from build123d import *

# Parameters (mm, degrees)
SKETCH1_W            = 210
SKETCH1_H            = 210
BASE_DEPTH           = 4
WALLS_START          = 4
SKETCH1_3_W          = 210
SKETCH1_3_H          = 210
SKETCH1_3_W_2        = 202
SKETCH1_3_H_2        = 202
WALLS_DEPTH          = 25.4
SCREWMOUNTS_DEPTH    = 25.4
SKETCH2_5_R          = 1.5
SCREWHOLES_DEPTH     = 12.5
ROUNDEDCORNERS_R     = 10
BACKHOLEMOUNTS_DEPTH = 4
SKETCH4_R            = 1.5
SKETCH4_W            = 30
SKETCH4_H            = 10
BATTERYPACK_DEPTH    = 4


with BuildPart() as part:
    # Sketch1 → Base (new body)
    with BuildSketch(Plane(origin=(0, 0, 0), x_dir=(1, 0, 0), z_dir=(0, 1, 0))):
        Rectangle(SKETCH1_W, SKETCH1_H)
    extrude(amount=BASE_DEPTH)

    # Sketch1<3> → Walls (add)
    with BuildSketch(Plane(origin=(0, 0, 0), x_dir=(1, 0, 0), z_dir=(0, 1, 0)).offset(WALLS_START)):
        Rectangle(SKETCH1_3_W, SKETCH1_3_H)
        Rectangle(SKETCH1_3_W_2, SKETCH1_3_H_2, mode=Mode.SUBTRACT)
    extrude(amount=WALLS_DEPTH)

    # Sketch2 → ScrewMounts (add)
    with BuildSketch(Plane(origin=(0, 29.4, 0), x_dir=(1, 0, 0), z_dir=(0, 1, 0))):
        with BuildLine():
            Line((-101, 101), (-101, 96))
            ThreePointArc((-101, 96), (-97.464466094, 97.464466094), (-96, 101))
            Line((-96, 101), (-101, 101))
        make_face()
        with BuildLine():
            Line((-101, -101), (-96, -101))
            ThreePointArc((-96, -101), (-97.464466094, -97.464466094), (-101, -96))
            Line((-101, -96), (-101, -101))
        make_face()
        with BuildLine():
            Line((101, 101), (96, 101))
            ThreePointArc((96, 101), (97.464466094, 97.464466094), (101, 96))
            Line((101, 96), (101, 101))
        make_face()
        with BuildLine():
            Line((101, -101), (101, -96))
            ThreePointArc((101, -96), (97.464466094, -97.464466094), (96, -101))
            Line((96, -101), (101, -101))
        make_face()
    extrude(amount=-SCREWMOUNTS_DEPTH)

    # Sketch2<5> → ScrewHoles (cut)
    with BuildSketch(Plane(origin=(0, 29.4, 0), x_dir=(1, 0, 0), z_dir=(0, 1, 0))):
        with Locations((-99.833273811, 99.833273811)):
            Circle(SKETCH2_5_R)
        with Locations((-99.833273811, -99.833273811)):
            Circle(SKETCH2_5_R)
        with Locations((99.833273811, 99.833273811)):
            Circle(SKETCH2_5_R)
        with Locations((99.833273811, -99.833273811)):
            Circle(SKETCH2_5_R)
    extrude(amount=-SCREWHOLES_DEPTH, mode=Mode.SUBTRACT)

    # RoundedCorners
    roundedcorners_edges = [part.edges().sort_by_distance(p)[0] for p in [
        (-105, 14.7, 105),
        (105, 14.7, 105),
        (105, 14.7, -105),
        (-105, 14.7, -105),
    ]]
    fillet(roundedcorners_edges, radius=ROUNDEDCORNERS_R)

    # Sketch3 → BackHoleMounts (cut)
    with BuildSketch(Plane.XZ):
        with BuildLine():
            Line((-77.985, 80), (-77.985, 61.974012195))
            ThreePointArc((-77.985, 61.974012195), (-75, 52.505), (-72.015, 61.974012195))
            Line((-72.015, 61.974012195), (-72.015, 80))
            ThreePointArc((-72.015, 80), (-75, 82.985), (-77.985, 80))
        make_face()
        with BuildLine():
            Line((77.985, 80), (77.985, 61.974012195))
            ThreePointArc((77.985, 61.974012195), (75, 52.505), (72.015, 61.974012195))
            Line((72.015, 61.974012195), (72.015, 80))
            ThreePointArc((72.015, 80), (75, 82.985), (77.985, 80))
        make_face()
        with BuildLine():
            Line((72.015, -70), (72.015, -88.025987805))
            ThreePointArc((72.015, -88.025987805), (75, -97.495), (77.985, -88.025987805))
            Line((77.985, -88.025987805), (77.985, -70))
            ThreePointArc((77.985, -70), (75, -67.015), (72.015, -70))
        make_face()
        with BuildLine():
            Line((-77.985, -70), (-77.985, -88.025987805))
            ThreePointArc((-77.985, -88.025987805), (-75, -97.495), (-72.015, -88.025987805))
            Line((-72.015, -88.025987805), (-72.015, -70))
            ThreePointArc((-72.015, -70), (-75, -67.015), (-77.985, -70))
        make_face()
    extrude(amount=-BACKHOLEMOUNTS_DEPTH, mode=Mode.SUBTRACT)

    # Sketch4 → BatteryPack (cut)
    with BuildSketch(Plane.XY.offset(105)):
        with Locations((75, 16.9)):
            Circle(SKETCH4_R)
        with Locations((-5, 16.9)):
            Circle(SKETCH4_R)
        with Locations((-50, 16.9)):
            Rectangle(SKETCH4_W, SKETCH4_H)
    extrude(amount=-BATTERYPACK_DEPTH, mode=Mode.SUBTRACT)


solid = part.part
Read the model definition and answer for the solid it produces. Units are mm, in the model's axes. A direction names the side the tool comes from. Give positions to 0.01 mm unless a question says otherwise; leave off trailing zeros. Write each loop counter-clockwise with the first axis right and the second up, starting at its lowest first coordinate (ties: lowest second). Pieces come first, ordered by that corner, then holes. Notation, with made-up numbers: (-10.5, 48.25) - (7.5, 48.25) arc R12 cw to (7.5, 68.25) - close; hole circle Ø7 at (23, 5.5). An arc over 180 degrees is marked (long way). Answer in a Markdown table with one row per item. Add a question column.
Item 1: Find the intervals of material crossed by L1, parallel to X at y = 2.3, z = 57.71 (3 decimals); L2, parallel to Z at x = -75, y = 2.3 (3 decimals); L3, parallel to Z at x = 39.5, y = 15, in increasing order.
Item 2: Section B-B, the plane z = 55.5 is taken. Write down the section's boundary in (x, y).
Item 3: Determine the mould class of faces 1 (the face through (-1, 14, -105)), 2 (the face through (-105, 14, 1)), 3 (the face through (-98, 17, -97)), 4 (the face through (-75.18, 1.97, -97.49)) for opening direction Z: pulls with the +Z half, pulls with the -Z half, needs draft (parallel to the pull), parting line crosses it, or undercut.
Item 4: Section D-D, the plane z = 20 is taken. Write down the section's boundary in (x, y).
Item 5: Section A-A, the plane x = -75 is taken. Write down the section's boundary in (y, z) (3 decimals), and give its area (3 significant figures).
Item 6: Section C-C, the plane x = 49 is taken. Write down the section's boundary in (y, z), and give its area (3 significant figures).
Item 7: A tool of negligible diameter and unlimited length cuts with its end or side. For faces 5 (the face through (-102, 29.4, -47)), 6 (the face through (101, 17, 1)), from which of +Z, -Z, +X, -X, +Y, -Y can it reach the whole face along a straight path? Write none if from no direction.
Item 8: Flat-ended cylindrical pins translate along their axes: P1, Ø12, axis at x = -75, z = 57.71, coming from the +Y side; P2, Ø2, axis at y = 16, z = 104, coming from the -X side. Find the tip coordinate at first contact, or state that the pin passes through.
Recorded:
| question | item | result |
|---|---|---|
| 1 | L1 | x = -105 to -80.205, -69.795 to 69.795, 80.205 to 105 |
| 1 | L2 | z = -105 to -97.495, -67.015 to 52.505, 82.985 to 105 |
| 1 | L3 | z = -105 to -101, 101 to 105 |
| 2 | outline | (-105, 0) - (-79.71, 0) - (-79.71, 4) - (-101, 4) - (-101, 29.4) - (-105, 29.4) - close; (-70.29, 0) - (70.29, 0) - (70.29, 4) - (-70.29, 4) - close; (79.71, 0) - (105, 0) - (105, 29.4) - (101, 29.4) - (101, 4) - (79.71, 4) - close |
| 3 | face 1 | pulls with the -Z half |
| 3 | face 2 | needs draft |
| 3 | face 3 | undercut |
| 3 | face 4 | undercut |
| 4 | outline | (-105, 0) - (105, 0) - (105, 29.4) - (101, 29.4) - (101, 4) - (-101, 4) - (-101, 29.4) - (-105, 29.4) - close |
| 5 | outline | (0, -105) - (29.4, -105) - (29.4, -101) - (4, -101) - (4, -97.495) - (0, -97.495) - close; (0, -67.015) - (4, -67.015) - (4, 52.505) - (0, 52.505) - close; (0, 82.985) - (4, 82.985) - (4, 101) - (29.4, 101) - (29.4, 105) - (0, 105) - close |
| 5 | area | 799 mm2 |
| 6 | outline | (0, -105) - (29.4, -105) - (29.4, -101) - (4, -101) - (4, 101) - (29.4, 101) - (29.4, 105) - (0, 105) - close |
| 6 | area | 1,040 mm2 |
| 7 | face 5 | +Z, -Z, +X, -X, +Y |
| 7 | face 6 | +Y |
| 8 | P1 | stops at y = 4 |
| 8 | P2 | stops at x = -101 |
